Input: part model. Units: mm. Frame: model coordinates. Face numbers are marked on the shaded views. Coordinates: 2 decimals unless noted, no trailing zeros. Order: outer loops, then holes, each group sorted by start corner. A loop starts at its lowest first (then second) coordinate and runs counter-clockwise, first axis right, second up. Notation, with made-up numbers: M -31,57.25 L 12,57.25 A16 cw 12,86.25 Z; hole C -20,-38.5 d3. An arc over 180 degrees is marked long. One line per item, written item: value.
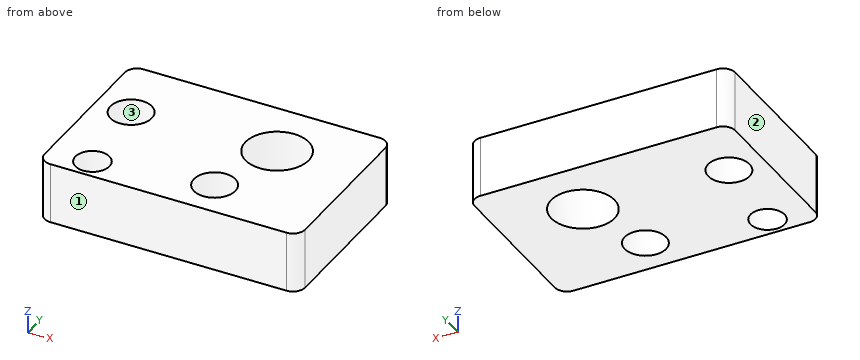
```python
from build123d import *

# Parameters (mm, degrees)
F0_W     = 106.902622
F0_H     = 71.619071
F1_DEPTH = 25
F2_R     = 5
F4_D     = 14
F5_D     = 17
F6_D     = 17
F7_D     = 26


with BuildPart() as f1:
    # F0 (on Top) → F1 (new body)
    with BuildSketch(Plane.XY):
        with Locations((8.139081, -35.809535)):
            Rectangle(F0_W, F0_H)
    extrude(amount=F1_DEPTH)

    # F2
    f2_edges = [f1.edges().sort_by_distance(p)[0] for p in [
        (-45.31223, -71.619071, 12.5),
        (61.590392, -71.619071, 12.5),
        (61.590392, 0, 12.5),
        (-45.31223, 0, 12.5),
    ]]
    fillet(f2_edges, radius=F2_R)

    # F4 (through all)
    with Locations(Plane.XY.offset(25)):
        with Locations((-27.718794, -62.822722)):
            Hole(F4_D / 2)

    # F5 (through all)
    with Locations(Plane.XY.offset(25)):
        with Locations((-30.82606, -27.311074)):
            Hole(F5_D / 2)

    # F6 (through all)
    with Locations(Plane.XY.offset(25)):
        with Locations((18.690022, -55.862375)):
            Hole(F6_D / 2)

    # F7 (through all)
    with Locations(Plane.XY.offset(25)):
        with Locations((28.00785, -25.314316)):
            Hole(F7_D / 2)


solid = f1.part
```
(1) Cut plane C-C on z = 16. Output: boundary loops of the cut face in (x, y), plus the area to 3 significant figures.
Data:
outline: M -45.31,-66.62 A5 ccw -40.31,-71.62 L 56.59,-71.62 A5 ccw 61.59,-66.62 L 61.59,-5 A5 ccw 56.59,0 L -40.31,0 A5 ccw -45.31,-5 Z; hole C -30.83,-27.31 d17; hole C -27.72,-62.82 d14; hole C 18.69,-55.86 d17; hole C 28.01,-25.31 d26
area: 6,500 mm2
(2) Cut plane A-A on x = 29.5. Output: boundary loops of the cut face in (y, z).
Data:
outline: M -71.62,0 L -38.23,0 L -38.23,25 L -71.62,25 Z; M -12.4,0 L 0,0 L 0,25 L -12.4,25 Z
(3) Cut plane B-B on y = -65.5. Output: boundary loops of the cut face in (x, z), plus the area to 3 significant figures.
Data:
outline: M -45.31,0 L -34.19,0 L -34.19,25 L -45.31,25 Z; M -21.25,0 L 61.59,0 L 61.59,25 L -21.25,25 Z
area: 2,350 mm2
(4) Draft query along Y for the marked faces 1, 2 and 3. Return one class per face: released by +Y, released by -Y, zero draft, split by the parting line, or undercut.
Data:
face 1: released by -Y
face 2: zero draft
face 3: undercut
(5) Ray query, line 1 (X direction, y = -26, z = 5.75); line 2 (X direction, y = -32.5, z = 5.25); line 3 (Y direction, x = -34, z = 18.5). Return the intervals inside material, ascending. Write a range as from..to.
Data:
line 1: x = -45.31..-39.22, -22.43..15.03, 40.99..61.59
line 2: x = -45.31..-37.56, -24.09..17.17, 38.84..61.59
line 3: y = -71.62..-65.91, -59.73..-35.2, -19.43..0
